Here's how the part is built. I have some questions about the finished solid (model axes, mm). A direction names the side the tool comes from. Round coordinates to 2 decimals unless told otherwise and drop trailing zeros. Write each loop counter-clockwise with the first axis right and the second up, starting at its lowest first coordinate (ties: lowest second). Pieces come first, ordered by that corner, then holes. Notation, with made-up numbers: (71.5, -28.75) -> (106.5, -28.75) arc R16 ccw to (106.5, -22.75) -> close; hole circle Ø3 at (-18, -38.5). An arc over 180 degrees is marked (long way). Answer in a Markdown table with one row per item.
from build123d import *

# Parameters (mm, degrees)
F0_W     = 304.8
F0_H     = 19.05
F1_DEPTH = 215.9
F2_W     = 279.4
F2_H     = 190.5
F3_DEPTH = 6.35
F4_R     = 6.35
F5_R     = 2.5
F6_DEPTH = 6.35


with BuildPart() as f1:
    # F0 (on Front) → F1 (new body)
    with BuildSketch(Plane.XZ):
        Rectangle(F0_W, F0_H)
    extrude(amount=F1_DEPTH)

    # F2 (on face) → F3 (cut)
    with BuildSketch(Plane(origin=(0, 0, -9.525), x_dir=(1, 0, 0), z_dir=(0, 0, -1))):
        with Locations((0, 107.95)):
            Rectangle(F2_W, F2_H)
    extrude(amount=-F3_DEPTH, mode=Mode.SUBTRACT)

    # F4
    f4_edges = [f1.edges().sort_by_distance(p)[0] for p in [
        (-152.4, -107.95, 9.525),
        (0, -215.9, 9.525),
        (152.4, -107.95, 9.525),
        (0, 0, 9.525),
    ]]
    fillet(f4_edges, radius=F4_R)

    # F5 (on face) → F6 (cut)
    with BuildSketch(Plane(origin=(0, 0, -9.525), x_dir=(1, 0, 0), z_dir=(0, 0, -1))):
        with Locations((127, 6.35)):
            Circle(F5_R)
        with Locations((-127, 6.35)):
            Circle(F5_R)
    extrude(amount=-F6_DEPTH, mode=Mode.SUBTRACT)


solid = f1.part
1) I want a section at B-B, the plane y = -66. List the corners of the cut face in (x, z) for me (3 decimals).
Response:
| item | result |
|---|---|
| outline | (-152.4, -9.525) -> (-139.7, -9.525) -> (-139.7, -3.175) -> (139.7, -3.175) -> (139.7, -9.525) -> (152.4, -9.525) -> (152.4, 3.175) arc R6.35 ccw to (146.05, 9.525) -> (-146.05, 9.525) arc R6.35 ccw to (-152.4, 3.175) -> close |
2) We'd pull the mould along X, two halves only. Please class faces 3 (the face through (-2, -109, -3.175)), 4 (the face through (-2, -215.9, -3)), 5 (the face through (-152.4, -106, -3)): +X half, -X half, draft (parallel to the pull), parting line (faces both ways), or undercut.
Response:
| item | result |
|---|---|
| face 3 | undercut |
| face 4 | draft |
| face 5 | -X half |
3) I want a section at A-A, the plane x = -55. List the corners of the cut face in (y, z) for me (3 decimals).
Response:
| item | result |
|---|---|
| outline | (-215.9, -9.525) -> (-203.2, -9.525) -> (-203.2, -3.175) -> (-12.7, -3.175) -> (-12.7, -9.525) -> (0, -9.525) -> (0, 3.175) arc R6.35 ccw to (-6.35, 9.525) -> (-209.55, 9.525) arc R6.35 ccw to (-215.9, 3.175) -> close |
4) I need wall thicknesses on line 1 (Y direction, x = -127, z = -5); line 2 (X direction, y = -6.35, z = -6); line 3 (X direction, y = -175, z = -5). Which ranges of each line are inside material? Lowest first, please. Write a range as [from, to].
Response:
| item | result |
|---|---|
| line 1 | y = [-215.9, -203.2], [-12.7, -8.85], [-3.85, 0] |
| line 2 | x = [-152.4, -129.5], [-124.5, 124.5], [129.5, 152.4] |
| line 3 | x = [-152.4, -139.7], [139.7, 152.4] |
5) Which directions (+Z, -Z, +X, -X, +Y, -Y) give clear straight access to the entire face, cutting with the end or side of a thin tool? Please do faces 1 (the face through (-150.589, -109.461, 7.615)), 2 (the face through (-139.7, -107, -6)).
Response:
| item | result |
|---|---|
| face 1 | +Z, -X, +Y, -Y |
| face 2 | -Z |
6) For pin 1 (3 mm diameter, centred on x = 127, y = -6.35, fed in from -Z) (3 decimals); pin 2 (1 mm diameter, centred on y = -122.5, z = 4.5, fed in from +X); pin 3 (1.5 mm diameter, centred on y = -173, z = 4.5, fed in from +X), each with a flat end and sliding along its axis, tell me the tip position at first contact or that it passes through.
Response:
| item | result |
|---|---|
| pin 1 | stops at z = -3.175 |
| pin 2 | stops at x = 152.35 |
| pin 3 | stops at x = 152.37 |
